For this review, take the finished solid that the model builds, in its own axes (mm). Face numbers are marked on the shaded views. Coordinates: 2 decimals unless noted, no trailing zeros. Write each loop counter-clockwise with the first axis right and the second up, starting at its lowest first coordinate (ties: lowest second). Pieces come first, ordered by that corner, then holes. Notation, with made-up numbers: (16.25, 58.5) -> (41.25, 58.5) arc R14 ccw to (41.25, 66.5) -> close; hole circle Ø9 at (33.5, 86.25). An arc over 180 degrees is marked (long way). Put each result on its own line as item: value. Start each with the question number.
Item 1: To check wall thickness, follow L1, parallel to Y at x = -20.5, z = 54.5; L2, parallel to Z at x = -3, y = -37. State the ranges of each line that lie inside material, in increasing order.
Item 2: Consider section B-B on x = -42. Give the boundary of the cut face in (y, z).
Item 3: Consider section A-A on z = -36. Give the boundary of the cut face in (x, y), and give its area (3 significant figures).
Item 4: The part is to be moulded in two halves that separate along X. For the marked faces 1, 2, 3 and 4, say which applies: +X half, -X half, draft (parallel to the pull), parting line (faces both ways), or undercut.
Item 5: Consider section C-C on x = 54.5. Give the boundary of the cut face in (y, z), and give its area (3 significant figures).
Item 6: Insertion check: P1, Ø3, axis at x = -22.5, z = -20.5, coming from the +Y side; P2, Ø3, axis at x = -24.5, y = -38, coming from the +Z side; P3, Ø1.1, axis at y = -38.5, z = -9, coming from the +X side. Each pin has a flat end and moves straight along its axis. Give the tip position at first contact, or say it passes through.
```python
from build123d import *

# Parameters (mm, degrees)
F0_W     = 152.824863
F0_H     = 135.844316
F1_DEPTH = 36.068
F2_W     = 120.878413
F2_H     = 101.30763
F2_R     = 6.390326
F2_R_2   = 6.098495
F3_DEPTH = 3.81


with BuildPart() as f1:
    # F0 (on Front) → F1 (new body)
    with BuildSketch(Plane.XZ):
        with Locations((-0.143901, -7.482948)):
            Rectangle(F0_W, F0_H)
    extrude(amount=F1_DEPTH)

    # F2 (on face) → F3 (join)
    with BuildSketch(Plane.XZ.offset(36.068)):
        with Locations((1.007318, -2.59025)):
            Rectangle(F2_W, F2_H)
        with Locations((-58.280665, -64.180687)):
            Circle(F2_R)
        with Locations((53.100161, -63.892879)):
            Circle(F2_R_2)
        with BuildLine():
            ThreePointArc((-20.616989, -59.863074), (-19.574403, -59.455771), (-19.139081, -58.42457))
            ThreePointArc((-19.139081, -58.42457), (-21.581818, -57.393368), (-20.616989, -59.863074))
        make_face()
        with BuildLine():
            ThreePointArc((-19.316033, -69.073379), (-19.755277, -67.992353), (-20.824042, -67.524063))
            ThreePointArc((-20.824042, -67.524063), (-21.976553, -70.154405), (-19.316033, -69.073379))
        make_face()
        with BuildLine():
            ThreePointArc((-8.490268, -67.922159), (-9.507815, -70.378735), (-7.051239, -69.361188))
            ThreePointArc((-7.051239, -69.361188), (-7.472721, -68.34364), (-8.490268, -67.922159))
        make_face()
        with BuildLine():
            ThreePointArc((-7.022742, -58.136765), (-9.527966, -57.099067), (-8.490268, -59.604292))
            ThreePointArc((-8.490268, -59.604292), (-7.45257, -59.174463), (-7.022742, -58.136765))
        make_face()
        with BuildLine():
            ThreePointArc((0, -59.378668), (1.08167, -58.930626), (1.529712, -57.848956))
            ThreePointArc((1.529712, -57.848956), (-1.08167, -56.767287), (0, -59.378668))
        make_face()
        with BuildLine():
            ThreePointArc((1.684347, -69.361188), (1.191013, -68.170175), (0, -67.676841))
            ThreePointArc((0, -67.676841), (-1.191013, -70.552201), (1.684347, -69.361188))
        make_face()
    extrude(amount=F3_DEPTH)


solid = f1.part
```
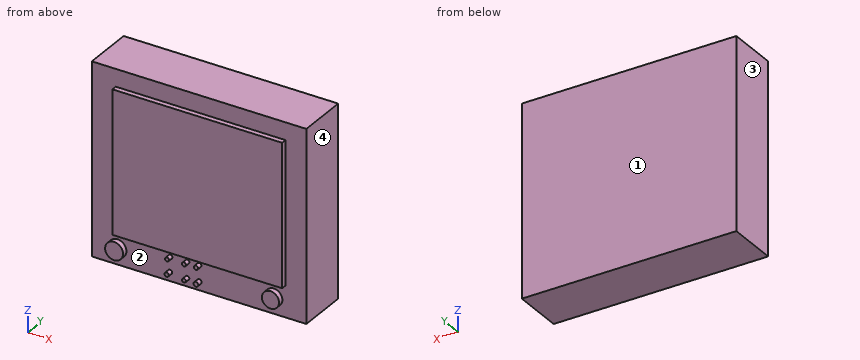
Return value:
1. L1: -36.07 to 0
1. L2: -53.24 to 48.06
2. outline: (-39.88, -53.24) -> (-36.07, -53.24) -> (-36.07, -75.41) -> (0, -75.41) -> (0, 60.44) -> (-36.07, 60.44) -> (-36.07, 48.06) -> (-39.88, 48.06) -> close
3. outline: (-76.56, -36.07) -> (-59.43, -36.07) -> (-59.43, -39.88) -> (61.45, -39.88) -> (61.45, -36.07) -> (76.27, -36.07) -> (76.27, 0) -> (-76.56, 0) -> close
3. area: 5,970 mm^2
4. face 1: draft
4. face 2: undercut
4. face 3: -X half
4. face 4: +X half
5. outline: (-39.88, -69.83) -> (-36.07, -69.83) -> (-36.07, -75.41) -> (0, -75.41) -> (0, 60.44) -> (-36.07, 60.44) -> (-36.07, 48.06) -> (-39.88, 48.06) -> (-39.88, -53.24) -> (-36.07, -53.24) -> (-36.07, -57.96) -> (-39.88, -57.96) -> close
5. area: 5,330 mm^2
6. P1: y = 0
6. P2: z = 48.06
6. P3: x = 61.45
